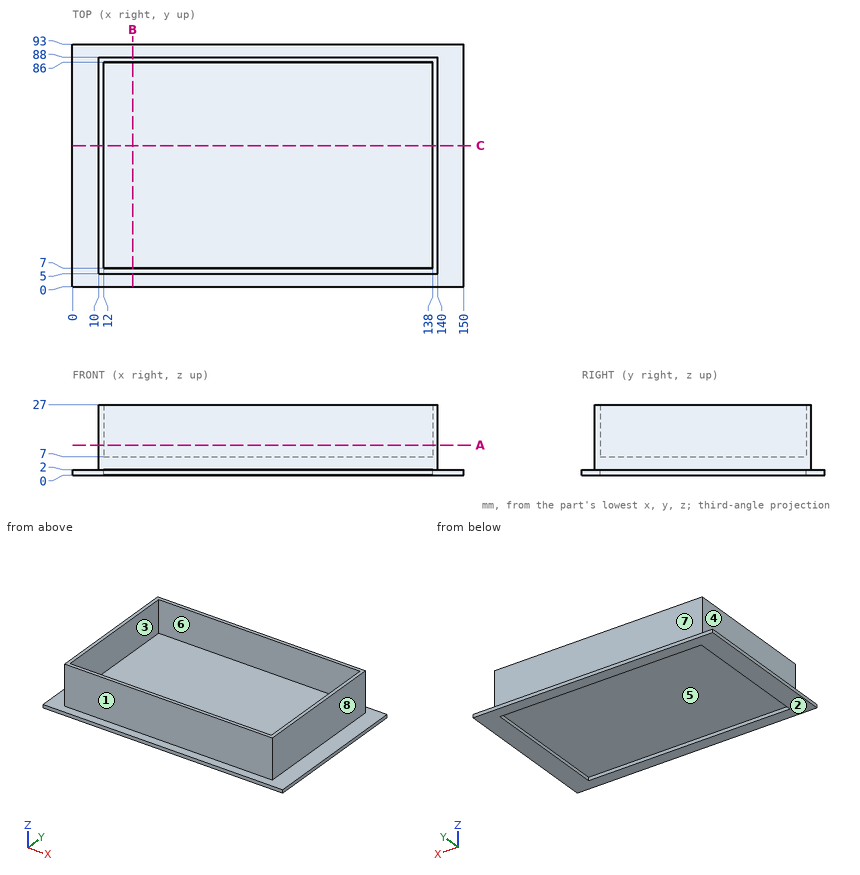
Verification items for this drawing (mm, ordinates from the low corner). A direction names the side the tool comes from. Coordinates: 2 decimals unless noted, no trailing zeros. Order: outer loops, then holes, each group sorted by start corner. A loop starts at its lowest first (then second) coordinate and runs counter-clockwise, first axis right, second up. Notation, with made-up numbers: M 53.25,46 L 74.25,46 A19 ccw 74.25,81 Z; hole C -25,-10 d4. An arc over 180 degrees is marked long. Use CSV: the item, a comma, the result in double quotes.
Item 1: Cross-section at B-B on x = 23. Record the cut outline in (y, z).
Returned:
outline,"M 0,0 L 7,0 L 7,2 L 86,2 L 86,0 L 93,0 L 93,2 L 88,2 L 88,27 L 86,27 L 86,7 L 7,7 L 7,27 L 5,27 L 5,2 L 0,2 Z"
Item 2: Gauge pin test, flat ends, axial feed: pin 1 Ø12 at (x, z) = (91, 22) entering from -Y; pin 2 Ø8 at (y, z) = (68.5, 4.5) entering from +X; pin 3 Ø7.5 at (y, z) = (37, 13.5) entering from +X; pin 4 Ø23.5 at (x, y) = (70.5, 46.5) entering from -Z. Record the tip position at first contact, or that the pin passes through.
Returned:
pin 1,"stops at y = 5"
pin 2,"stops at x = 150"
pin 3,"stops at x = 140"
pin 4,"stops at z = 2"
Item 3: Mould release check, pull along Y, two halves, no side actions. Record for the marked faces 1, 2 and 3: pulls with the +Y half, pulls with the -Y half, needs draft (parallel to the pull), parting line crosses it, or undercut.
Returned:
face 1,"pulls with the -Y half"
face 2,"needs draft"
face 3,"undercut"
Item 4: Cross-section at A-A on z = 11.5. Record the cut outline in (x, y), then the cut area to 3 significant figures.
Returned:
outline,"M 10,5 L 140,5 L 140,88 L 10,88 Z; hole M 12,7 L 138,7 L 138,86 L 12,86 Z"
area,"836 mm2"
Item 5: Thickness scan on line 1 along Y through (x, z) = (20, 22.5); line 2 along X through (y, z) = (43.5, 20.5); line 3 along Z through (x, y) = (44, 89). Record the ranges inside material, lowest first.
Returned:
line 1,"y = 5 to 7, 86 to 88"
line 2,"x = 10 to 12, 138 to 140"
line 3,"z = 0 to 2"
Item 6: Cross-section at C-C on y = 54. Record the cut outline in (x, z).
Returned:
outline,"M 0,0 L 12,0 L 12,2 L 138,2 L 138,0 L 150,0 L 150,2 L 140,2 L 140,27 L 138,27 L 138,7 L 12,7 L 12,27 L 10,27 L 10,2 L 0,2 Z"
Item 7: Tool access check on the marked faces 4, 5, 6, 7 and 8. Record the directions out of +Z, -Z, +X, -X, +Y, -Y that give a thin tool (end or side, any length) a straight path to the whole face; none if there is none.
Returned:
face 4,"+Z, -X, +Y, -Y"
face 5,"-Z"
face 6,"+Z"
face 7,"+Z, +X, -X, +Y"
face 8,"+Z, +X, +Y, -Y"
